Input: part model. Units: mm. Frame: model coordinates. Face numbers are marked on the shaded views. A direction names the side the tool comes from. Coordinates: 2 decimals unless noted, no trailing zeros. Write each loop counter-clockwise with the first axis right and the second up, starting at its lowest first coordinate (ties: lowest second). Pieces come first, ordered by that corner, then holes. Notation, with made-up numbers: M -22,17 L 8,17 A25 ccw 8,35 Z; hole C 33.5,40 d4. An arc over 180 degrees is marked long. Answer as a JSON object with one key per item and string values. Group by question number.
from build123d import *

# Parameters (mm, degrees)
SKETCH1_W           = 20
SKETCH1_H           = 20
BOSS_EXTRUDE1_DEPTH = 15
SKETCH2_W           = 12
SKETCH2_H           = 12
CUT_EXTRUDE1_DEPTH  = 9
SKETCH3_W           = 3
SKETCH3_H           = 2
CUT_EXTRUDE2_DEPTH  = 15
SKETCH4_W           = 3
SKETCH4_H           = 2
CUT_EXTRUDE3_DEPTH  = 15
SKETCH5_R           = 1.5
CUT_EXTRUDE4_DEPTH  = 15
SKETCH6_R           = 2.5
CUT_EXTRUDE5_DEPTH  = 12
CUT_EXTRUDE6_DEPTH  = 3
CUT_EXTRUDE7_DEPTH  = 3
CUT_EXTRUDE8_DEPTH  = 3


with BuildPart() as part:
    # Sketch1 → Boss-Extrude1 (new body)
    with BuildSketch(Plane(origin=(0, 0, 0), x_dir=(1, 0, 0), z_dir=(0, 1, 0))):
        with Locations((10, 10)):
            Rectangle(SKETCH1_W, SKETCH1_H)
    extrude(amount=BOSS_EXTRUDE1_DEPTH)

    # Sketch2 → Cut-Extrude1 (cut)
    with BuildSketch(Plane(origin=(0, 15, 0), x_dir=(1, 0, 0), z_dir=(0, 1, 0))):
        with Locations((6, 6)):
            Rectangle(SKETCH2_W, SKETCH2_H)
    extrude(amount=-CUT_EXTRUDE1_DEPTH, mode=Mode.SUBTRACT)

    # Sketch3 → Cut-Extrude2 (cut)
    with BuildSketch(Plane.XY):
        with Locations((13.5, 7)):
            Rectangle(SKETCH3_W, SKETCH3_H)
    extrude(amount=-CUT_EXTRUDE2_DEPTH, mode=Mode.SUBTRACT)

    # Sketch4 → Cut-Extrude3 (cut)
    with BuildSketch(Plane.ZY):
        with Locations((-13.5, 7)):
            Rectangle(SKETCH4_W, SKETCH4_H)
    extrude(amount=-CUT_EXTRUDE3_DEPTH, mode=Mode.SUBTRACT)

    # Sketch5 → Cut-Extrude4 (cut)
    with BuildSketch(Plane(origin=(0, 15, 0), x_dir=(1, 0, 0), z_dir=(0, 1, 0))):
        with Locations(Location((11, 11, 0), (0, 0, 270))):
            Circle(SKETCH5_R)
        with Locations(Location((17, 17, 0), (0, 0, 270))):
            Circle(SKETCH5_R)
    extrude(amount=-CUT_EXTRUDE4_DEPTH, mode=Mode.SUBTRACT)

    # Sketch6 → Cut-Extrude5 (cut)
    with BuildSketch(Plane(origin=(0, 15, 0), x_dir=(1, 0, 0), z_dir=(0, 1, 0))):
        with Locations(Location((11, 11, 0), (0, 0, 270))):
            Circle(SKETCH6_R)
    extrude(amount=-CUT_EXTRUDE5_DEPTH, mode=Mode.SUBTRACT)

    # Sketch7 → Cut-Extrude6 (cut)
    with BuildSketch(Plane(origin=(0, 0, 0), x_dir=(-1, 0, 0), z_dir=(0, -1, 0))):
        Polygon((-19.1, 14.71964915), (-16.075158234, 14.041171227), (-13.975158234, 16.321522077), (-14.9, 19.28035085), (-17.924841766, 19.958828773), (-20.024841766, 17.678477923), align=None)
    extrude(amount=-CUT_EXTRUDE6_DEPTH, mode=Mode.SUBTRACT)

    # Sketch8 → Cut-Extrude7 (cut)
    with BuildSketch(Plane(origin=(0, 0, 0), x_dir=(-1, 0, 0), z_dir=(0, -1, 0))):
        Polygon((-20, 14.71964915), (-19.1, 14.71964915), (-14.9, 19.28035085), (-14.9, 20), (-20, 20), align=None)
    extrude(amount=-CUT_EXTRUDE7_DEPTH, mode=Mode.SUBTRACT)

    # Sketch9 → Cut-Extrude8 (cut)
    with BuildSketch(Plane(origin=(0, 0, 0), x_dir=(-1, 0, 0), z_dir=(0, -1, 0))):
        Polygon((-13.673474415, 16.296986821), (-14.727909935, 19.529349074), (-14.727909935, 20), (-18.05443552, 20.232362253), (-20.326525585, 17.703013179), (-20.94475972, 14.470650926), (-19.272090065, 14.470650926), (-15.94556448, 13.767637747), align=None)
    extrude(amount=-CUT_EXTRUDE8_DEPTH, mode=Mode.SUBTRACT)


solid = part.part
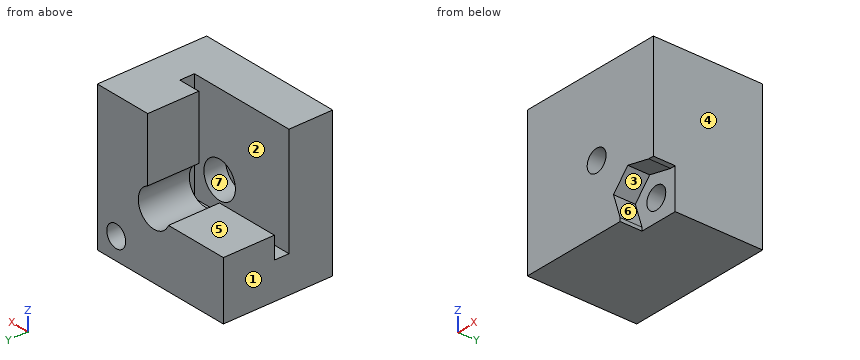
Q1. Section A-A, the plane x = 11. Return the cut outline in (y, z), and give its area (4 significant figures).
Q2. Draft query along X for the marked faces 1, 2, 3 and 4. Return one class per face: released by +X, released by -X, zero draft, split by the parting line, or undercut.
Q3. Access query for the marked faces 5, 6 and 7. Directions: +Z, -Z, +X, -X, +Y, -Y. A direction counts if a zero-diameter tool reaches every point of the face in a straight line with its end or side. Return the directions, or none.
Q4. Section D-D, the plane x = 4.5. Return the cut outline in (y, z), and give its area (3 significant figures).
Q5. Section C-C, the plane z = -11. Return the cut outline in (x, y).
Q6. Line query: line 1 (Y direction, x = 5, z = -14); line 2 (Z direction, x = 17, y = 5.25); line 3 (X direction, y = 8.5, z = -17). Output: solid intervals per line, ascending. Write a range as from..to.
Q7. Section B-B, the plane y = 10.5. Return the cut outline in (x, z), and give its area (3 significant figures).
Q8. Pin query (flat end, axial travel): pin 1 Ø0.8 at (x, y) = (19.5, 2) entering from -Z; pin 2 Ø10 at (x, z) = (11, -5) entering from +Y; pin 3 Ø2.5 at (x, z) = (12, -11) entering from +Y; pin 4 Ø0.6 at (x, y) = (7, 7) entering from +Z. Return the tip coordinate at first contact, or that it passes through.
Filled in:
{
 "1": {"outline": "M 0,-20 L 15,-20 L 15,-13.5 L 8,-13.5 L 8,-15 L 6,-15 L 6,-13.5 L 3,-13.5 L 3,-12.5 L 0,-12.5 Z; M 0,-9.5 L 3,-9.5 L 3,-8.5 L 6,-8.5 L 6,0 L 0,0 Z", "area": "151.5 mm^2"},
 "2": {"face 1": "released by -X", "face 2": "zero draft", "face 3": "undercut", "face 4": "released by +X"},
 "3": {"face 5": "+Z, -X, +Y", "face 6": "+X, -Y", "face 7": "+Y"},
 "4": {"outline": "M 0,-20 L 15,-20 L 15,-12 L 8,-12 L 8,-15 L 6,-15 L 6,0 L 0,0 Z", "area": "186 mm^2"},
 "5": {"outline": "M 0,0 L 9.5,0 L 9.5,3 L 8.5,3 L 8.5,6 L 0,6 Z; M 12.5,0 L 20,0 L 20,15 L 13.5,15 L 13.5,8 L 15,8 L 15,6 L 13.5,6 L 13.5,3 L 12.5,3 Z"},
 "6": {"line 1": "0..6, 8..15", "line 2": "-20..-18.5, -15.5..0", "line 3": "0..15.5, 18.5..20"},
 "7": {"outline": "M 0,-20 L 20,-20 L 20,0 L 12,0 L 12,-8.71 A2.5 cw long 8.71,-12 L 0,-12 Z; hole C 17,-17 d3", "area": "240 mm^2"},
 "8": {"pin 1": "z = -14.47", "pin 2": "y = 15", "pin 3": "y = 3", "pin 4": "z = -15"}
}
